Part model, mm, in its own coordinate system. Face numbers are marked on the shaded views. A direction names the side the tool comes from. Coordinates: 2 decimals unless noted, no trailing zeros. Write each loop counter-clockwise with the first axis right and the second up, starting at its lowest first coordinate (ties: lowest second). Pieces come first, ordered by that corner, then holes. Notation, with made-up numbers: (22, 12) -> (46, 12) arc R13 cw to (46, 20) -> close; hole circle Ø9 at (33.5, 25.25). An arc over 180 degrees is marked (long way). Write item = value, one per line. Start each with the question number.
Q1. Band-saw the part on D-D, the plane y = 7. List the corners of the cut face in (x, z) (3 decimals).
Q2. Band-saw the part on C-C, the plane x = 4. List the corners of the cut face in (y, z) (3 decimals).
Q3. Probe line 1 (Z direction, x = 0, y = 0.2) (1 decimal); line 2 (Z direction, x = -1, y = -8.75); line 3 (Y direction, x = 1.75, z = -18). List the from-to ranges inside material, lowest first.
Q4. Pin check, flat tips, straight feed: P1, Ø6, axis at x = -2.5, y = 5.5, coming from the -Z side; P2, Ø1.5, axis at x = 1, z = 7.5, coming from the -Y side; P3, Ø5, axis at x = -1.5, y = -13.5, coming from the +Z side; P4, Ø1.1, axis at x = 0, z = 9.05, coming from the +Y side. Stop position of each tip, or through.
Q5. Band-saw the part on B-B, the plane z = 0. List the corners of the cut face in (x, y) (3 decimals), plus the area to 3 significant figures.
Q6. Tool access for the marked faces 1, 2, 3, 4 and 5: list every direction of +Z, -Z, +X, -X, +Y, -Y with a clear straight run to the whole face (end or side of a thin tool).
Q7. Band-saw the part on A-A, the plane x = 0. Give the number of separate pieces and of enclosed holes in the cut face, plus the area to 3 significant figures.
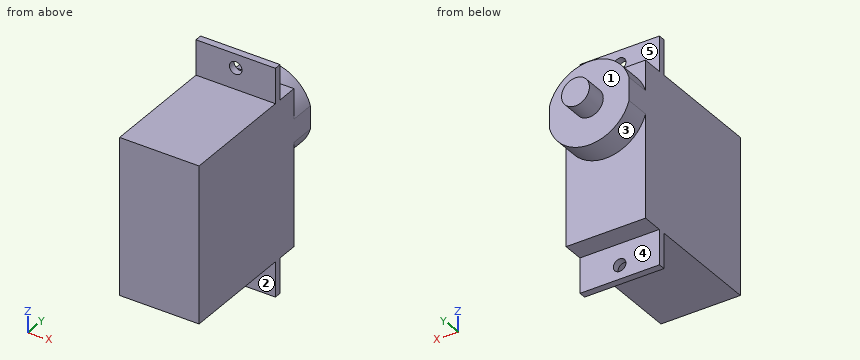
Autodesk Inventor part; units mm, degrees
ref_plane "YZ Plane" through (0, 0, 0) normal (1, 0, 0) x (0, 1, 0)
ref_plane "XZ Plane" through (0, 0, 0) normal (0, 1, 0) x (-1, 0, 0)
ref_plane "XY Plane" through (0, 0, 0) normal (0, 0, 1) x (1, 0, 0)
sketch "Sketch1" plane through (0, 0, 0) normal (0, 1, 0) x (-1, 0, 0)
  line L0 (-5.705, 6) -> (5.705, 6)
  line L1 (5.705, 6) -> (5.705, -16.48)
  line L2 (5.705, -16.48) -> (-5.705, -16.48)
  line L3 (-5.705, -16.48) -> (-5.705, 6)
  line L4 (-5.705, 11.035) -> (5.705, 11.035)
  line L5 (5.705, 11.035) -> (5.705, -21.515)
  line L6 (5.705, -21.515) -> (-5.705, -21.515)
  line L7 (-5.705, -21.515) -> (-5.705, 11.035)
  circle A0 centre (0, 0) radius 2
  line L8 (0, 9.0475) -> (0, 11.035) construction
  line L9 (0, -19.5275) -> (0, -21.515) construction
  line L10 (-5.705, 6) -> (-5.705, 11.035) construction
  line L11 (-5.705, -16.48) -> (-5.705, -21.515) construction
  arc A1 (5.705, 1.6543) -> (-5.705, 1.6543) centre (0, 0) ccw
  arc A2 (-5.705, -1.6543) -> (5.705, -1.6543) centre (0, 0) ccw
  line L12 (5.705, 11.035) -> (-5.705, 11.035)
  line L13 (-5.705, 11.035) -> (-5.705, 6)
  line L14 (-5.705, 6) -> (5.705, 6)
  line L15 (5.705, 6) -> (5.705, 11.035)
  line L16 (5.705, -16.48) -> (-5.705, -16.48)
  line L17 (-5.705, -16.48) -> (-5.705, -21.515)
  line L18 (-5.705, -21.515) -> (5.705, -21.515)
  line L19 (5.705, -21.515) -> (5.705, -16.48)
  point P0 (0, 6)
  dimension "d0" = 11.41
  dimension "d8" = 32.55
  dimension "d10" = 4
  dimension "d28" = 22.48
  dimension "d29" = 6
  dimension "d30" = 28.575
  dimension "d31" = 5.94
extrude "Extrusion1" add sketch "Sketch1" along normal blind 4 and the other way blind 16.52 contours L0 L1 A1 L3 | A1 L1 A2 L3 | A2 L1 L2 L3 | A0
extrude "Extrusion5" add sketch "Sketch1" along normal blind 1 contours L7 L4 L5 L0 | L2 L5 L6 L7
extrude "Extrusion3" add sketch "Sketch1" along normal blind 7.56 contours A1 L1 A2 L3
extrude "Extrusion4" add sketch "Sketch1" along normal blind 10.56 contours A0
hole "Hole1" at (0, 0, 9.0475) at (0, 0, -19.5275) direction (0, 1, 0) diameter 1.8 end through all
properties part number "HS55"
Ans:
q1.outline = (-5.705, -1.654) arc R5.94 ccw to (5.705, -1.654) -> (5.705, 1.654) arc R5.94 ccw to (-5.705, 1.654) -> close
q2.outline = (-16.52, -16.48) -> (0, -16.48) -> (0, -21.515) -> (1, -21.515) -> (1, -16.48) -> (4, -16.48) -> (4, -4.391) -> (7.56, -4.391) -> (7.56, 4.391) -> (4, 4.391) -> (4, 6) -> (1, 6) -> (1, 11.035) -> (0, 11.035) -> (0, 6) -> (-16.52, 6) -> close
q3.line_1 = -21.5 to -20.4, -18.6 to 8.1, 9.9 to 11
q3.line_2 = -16.48 to 6
q3.line_3 = 0 to 1
q4.P1 = -16.48
q4.P2 = 0
q4.P3 = 6
q4.P4 = through
q5.outline = (-5.705, -16.52) -> (5.705, -16.52) -> (5.705, 7.56) -> (2, 7.56) -> (2, 10.56) -> (-2, 10.56) -> (-2, 7.56) -> (-5.705, 7.56) -> close
q5.area = 287 mm2
q6.face_1 = +Y
q6.face_2 = -Z, +X, -X, -Y
q6.face_3 = -Z, +Y
q6.face_4 = -Z, +X, -X, +Y
q6.face_5 = +Z, +X, -X, +Y
q7.separate_pieces = 3
q7.enclosed_holes = 0
q7.area = 522 mm2
